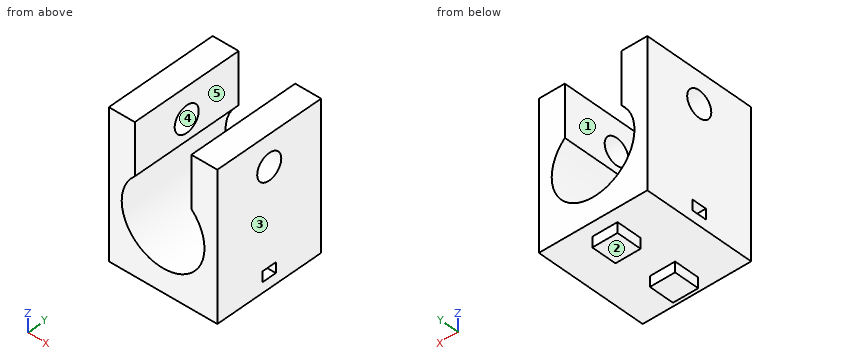
```python
from build123d import *

# Parameters (mm, degrees)
BOSS_EXTRUDE1_DEPTH = 11
CUT_EXTRUDE1_REACH  = 30.128
SKETCH2_R           = 2.55
SKETCH4_W           = 2
SKETCH4_H           = 2.8
CUT_EXTRUDE3_DEPTH  = 21.1
SKETCH5_W           = 4.9
SKETCH5_H           = 4.9
BOSS_EXTRUDE2_DEPTH = 2


with BuildPart() as part:
    # Sketch1 → Boss-Extrude1 (new, symmetric)
    with BuildSketch(Plane(origin=(0, 0, 0), x_dir=(1, 0, 0), z_dir=(0, 1, 0))):
        with BuildLine():
            Line((-5.5, -15), (-10.55, -15))
            Line((-10.55, -15), (-10.55, 13.42813746))
            Line((-10.55, 13.42813746), (10.55, 13.42813746))
            Line((10.55, 13.42813746), (10.55, -15))
            Line((10.55, -15), (5.5, -15))
            Line((5.5, -15), (5.5, -5))
            ThreePointArc((5.5, -5), (0, 8.92813746), (-5.5, -5))
            Line((-5.5, -5), (-5.5, -15))
        make_face()
    extrude(amount=BOSS_EXTRUDE1_DEPTH, both=True)

    # Cut-Extrude1: up to this face of the body (flat: up to its plane)
    cut_extrude1_end = Plane(part.part.faces().sort_by_distance((-10.55, 0, 0.78593127))[0])
    # Sketch2 → Cut-Extrude1 (cut, up to the picked face)
    with BuildSketch(Plane(origin=(10.55, 0, 0), x_dir=(0, 0, -1), z_dir=(1, 0, 0)), mode=Mode.PRIVATE) as cut_extrude1_sk1:
        with Locations((-9, 0)):
            Circle(SKETCH2_R)
    cut_extrude1_tool1 = split(extrude(cut_extrude1_sk1.sketch, amount=-CUT_EXTRUDE1_REACH, mode=Mode.PRIVATE), bisect_by=cut_extrude1_end, keep=Keep.BOTH, mode=Mode.PRIVATE)
    add(cut_extrude1_tool1.solids().sort_by(Axis((10.55, 0, 9), (-1, 0, 0)))[0], mode=Mode.SUBTRACT)

    # Sketch4 → Cut-Extrude3 (cut)
    with BuildSketch(Plane(origin=(10.55, 0, 0), x_dir=(0, 0, -1), z_dir=(1, 0, 0))):
        with Locations((10.42813746, 0)):
            Rectangle(SKETCH4_W, SKETCH4_H)
    extrude(amount=-CUT_EXTRUDE3_DEPTH, mode=Mode.SUBTRACT)

    # Sketch5 → Boss-Extrude2 (add)
    with BuildSketch(Plane(origin=(0, 0, -13.42813746), x_dir=(-1, 0, 0), z_dir=(0, 0, -1))):
        with Locations((0.05, 6.1)):
            Rectangle(SKETCH5_W, SKETCH5_H)
        with Locations((0.05, -6.1)):
            Rectangle(SKETCH5_W, SKETCH5_H)
    extrude(amount=BOSS_EXTRUDE2_DEPTH)


solid = part.part
```
The model under review builds one solid part; all positions refer to its coordinate system, in mm. Face numbers are marked on the shaded views. A direction names the side the tool comes from. Give positions to 0.01 mm unless a question says otherwise; leave off trailing zeros. Write each loop counter-clockwise with the first axis right and the second up, starting at its lowest first coordinate (ties: lowest second). Pieces come first, ordered by that corner, then holes. Notation, with made-up numbers: (46.5, -35) - (97.5, -35) arc R20 cw to (97.5, -20) - close; hole circle Ø8 at (-6.75, 41.5). An arc over 180 degrees is marked (long way). Answer in a Markdown table with one row per item. Add a question column.
1. We need section C-C on y = 0. Write out the cut boundary in (x, z), then the cut area to 3 significant figures.
2. We need section D-D on z = 9. Write out the cut boundary in (x, y).
3. We need section B-B on z = -10.5. Write out the cut boundary in (x, y), then the cut area to 3 significant figures.
4. We need section A-A on x = -6.25. Write out the cut boundary in (y, z).
5. Tool access review of the marked faces 4 and 5: name each direction out of +Z, -Z, +X, -X, +Y, -Y from which nothing blocks a thin tool from reaching the whole face with its end or side.
6. Draft analysis for pull direction X (two halves, no side actions). For the marked faces 1, 2 and 3, state which applies: +X half, -X half, draft (parallel to the pull), parting line (faces both ways), or undercut.
7. Wall thickness on line 1 along X through (y, z) = (-2.5, 10); line 2 along X through (y, z) = (9.25, -1); line 3 along Y through (x, z) = (-7.85, 9): over which ranges is each line inside the solid? List them lowest first. Write a range as [from, to].
8. Insertion check: P1, Ø0.6, axis at x = -0.5, z = -14.5, coming from the -Y side; P2, Ø4, axis at y = 0, z = 9, coming from the -X side; P3, Ø1, axis at y = 5.5, z = -14, coming from the -X side; P4, Ø1, axis at x = -1, z = -15, coming from the +Y side. Each pin has a flat end and moves straight along its axis. Give the tip position at first contact, or say it passes through.
Ans:
| question | item | result |
|---|---|---|
| 1 | outline | (-10.55, -13.43) - (10.55, -13.43) - (10.55, -11.43) - (-10.55, -11.43) - close; (-10.55, -9.43) - (10.55, -9.43) - (10.55, 6.45) - (5.5, 6.45) - (5.5, 5) arc R8.05 cw (long way) to (-5.5, 5) - (-5.5, 6.45) - (-10.55, 6.45) - close; (-10.55, 11.55) - (-5.5, 11.55) - (-5.5, 15) - (-10.55, 15) - close; (5.5, 11.55) - (10.55, 11.55) - (10.55, 15) - (5.5, 15) - close |
| 1 | area | 209 mm^2 |
| 2 | outline | (-10.55, -11) - (-5.5, -11) - (-5.5, -2.55) - (-10.55, -2.55) - close; (-10.55, 2.55) - (-5.5, 2.55) - (-5.5, 11) - (-10.55, 11) - close; (5.5, -11) - (10.55, -11) - (10.55, -2.55) - (5.5, -2.55) - close; (5.5, 2.55) - (10.55, 2.55) - (10.55, 11) - (5.5, 11) - close |
| 3 | outline | (-10.55, -11) - (10.55, -11) - (10.55, -1.4) - (-10.55, -1.4) - close; (-10.55, 1.4) - (10.55, 1.4) - (10.55, 11) - (-10.55, 11) - close |
| 3 | area | 405 mm^2 |
| 4 | outline | (-11, -13.43) - (11, -13.43) - (11, -5.95) - (-11, -5.95) - close; (-11, 4.2) - (11, 4.2) - (11, 15) - (-11, 15) - close; hole circle Ø5.1 at (0, 9); hole (-1.4, -11.43) - (1.4, -11.43) - (1.4, -9.43) - (-1.4, -9.43) - close |
| 5 | face 4 | +X, -X |
| 5 | face 5 | +Z, +Y, -Y |
| 6 | face 1 | undercut |
| 6 | face 2 | draft |
| 6 | face 3 | +X half |
| 7 | line 1 | x = [-10.55, -5.5], [5.5, 10.55] |
| 7 | line 2 | x = [-10.55, -8.05], [8.05, 10.55] |
| 7 | line 3 | y = [-11, -2.55], [2.55, 11] |
| 8 | P1 | stops at y = -8.55 |
| 8 | P2 | passes through |
| 8 | P3 | stops at x = -2.5 |
| 8 | P4 | stops at y = 8.55 |
